```python
from build123d import *

# Parameters (mm, degrees)
PAD_DEPTH       = 8
PAD001_DEPTH    = 4
POCKET_DEPTH    = 5
SKETCH003_W     = 13
SKETCH003_H     = 7
PAD002_DEPTH    = 1
SKETCH004_R     = 0.5
POCKET001_DEPTH = 13.001
PAD003_DEPTH    = 14
PAD004_DEPTH    = 14
SKETCH007_R     = 1.5
PAD005_DEPTH    = 6
POCKET002_DEPTH = 5
SKETCH009_R     = 3
POCKET003_DEPTH = 15
SKETCH010_W     = 190
SKETCH010_H     = 10
POCKET004_DEPTH = 10
SKETCH011_W     = 40
SKETCH011_H     = 13
POCKET005_DEPTH = 3
PAD006_DEPTH    = 14
SKETCH014_W     = 25
SKETCH014_H     = 9
POCKET006_DEPTH = 15
SKETCH015_W     = 19.00002
SKETCH015_H     = 12
PAD007_DEPTH    = 1
SKETCH016_W     = 50
SKETCH016_H     = 9
PAD008_DEPTH    = 1
SKETCH017_W     = 3.141787
SKETCH017_H     = 1.901607
PAD009_DEPTH    = 2
SKETCH018_W     = 15
SKETCH018_H     = 8
POCKET007_DEPTH = 5
SKETCH019_W     = 4.140358
SKETCH019_H     = 3.938392
PAD010_DEPTH    = 1
FILLET_R        = 4


with BuildPart() as part:
    # Sketch → Pad (new body)
    with BuildSketch(Plane.XY):
        with BuildLine():
            Line((107.5, 0), (107.5, -35))
            Line((107.5, -35), (-107.5, -35))
            Line((-107.5, -35), (-107.5, 0))
            Line((-107.5, 0), (-0.930233, -9.956639))
            ThreePointArc((-0.930233, -9.956639), (0, -10), (0.930233, -9.956639))
            Line((0.930233, -9.956639), (107.5, 0))
        make_face()
    extrude(amount=PAD_DEPTH)

    # Sketch001 (on Face8 of Pad) → Pad001 (join)
    with BuildSketch(Plane.XY.offset(8)):
        with BuildLine():
            Line((107.5, 0), (107.5, -35))
            Line((107.5, -35), (-107.5, -35))
            Line((-107.5, -35), (-107.5, 0))
            Line((-107.5, 0), (-15, 0))
            Line((-15, 0), (-15, 2))
            ThreePointArc((15, 2), (0, 17), (-15, 2))
            Line((15, 2), (15, 0))
            Line((15, 0), (107.5, 0))
        make_face()
    extrude(amount=PAD001_DEPTH)

    # Sketch002 (on Face12 of Pad001) → Pocket (cut)
    with BuildSketch(Plane.XY.offset(12)):
        with BuildLine():
            ThreePointArc((3, -5.196152), (0, 6), (-3, -5.196152))
            Line((-3, -5.196152), (-3, -6.5))
            ThreePointArc((-3, -6.5), (0, -9.5), (3, -6.5))
            Line((3, -5.196152), (3, -6.5))
        make_face()
    extrude(amount=-POCKET_DEPTH, mode=Mode.SUBTRACT)

    # Sketch003 (on Face12 of Pocket) → Pad002 (join)
    with BuildSketch(Plane.XY.offset(12)):
        with Locations((0, 10)):
            Rectangle(SKETCH003_W, SKETCH003_H)
        with Locations((0, -20)):
            Rectangle(SKETCH003_W, SKETCH003_H)
    extrude(amount=PAD002_DEPTH)

    # Sketch004 (on Face31 of Pad002) → Pocket001 (cut, through all)
    with BuildSketch(Plane.XY.offset(13)):
        with Locations((0, 8.75)):
            Circle(SKETCH004_R)
        with Locations((0, -19.25)):
            Circle(SKETCH004_R)
    extrude(amount=-POCKET001_DEPTH, mode=Mode.SUBTRACT)

    # Sketch005 (on Face13 of Pocket001) → Pad003 (join)
    with BuildSketch(Plane.XY.offset(12)):
        with BuildLine():
            ThreePointArc((-6.5, 13.5), (-8.621333, 12.621327), (-9.50002, 10.5))
            Line((-9.50002, 10.5), (-9.50002, -20.5))
            ThreePointArc((-9.50002, -20.5), (-8.621333, -22.621327), (-6.5, -23.5))
            Line((-6.5, -23.5), (-6.5, 13.5))
        make_face()
        with BuildLine():
            ThreePointArc((6.5, -23.5), (8.62132, -22.62132), (9.5, -20.5))
            Line((9.5, 10.5), (9.5, -20.5))
            ThreePointArc((9.5, 10.5), (8.62132, 12.62132), (6.5, 13.5))
            Line((6.5, 13.5), (6.5, -23.5))
        make_face()
    extrude(amount=PAD003_DEPTH)

    # Sketch006 (on Face13 of Pad003) → Pad004 (join)
    with BuildSketch(Plane.XY.offset(12)):
        with BuildLine():
            Line((-107.5, 0), (-15, 0))
            Line((-15, 0), (-15, 2))
            ThreePointArc((15, 2), (0, 17), (-15, 2))
            Line((15, 0), (15, 2))
            Line((15, 0), (107.5, 0))
            Line((107.5, 0), (107.5, -2))
            Line((107.5, -2), (13, -2))
            Line((13, 2), (13, -2))
            ThreePointArc((13, 2), (0, 15), (-13, 2))
            Line((-13, 2), (-13, -2))
            Line((-13, -2), (-107.5, -2))
            Line((-107.5, -2), (-107.5, 0))
        make_face()
    extrude(amount=PAD004_DEPTH)

    # Sketch007 (on Face14 of Pad004) → Pad005 (join)
    with BuildSketch(Plane.XY.offset(12)):
        with BuildLine():
            ThreePointArc((-107.5, -5.999985), (-100.671578, -8.828432), (-103.5, -2))
            Line((-103.5, -2), (-107.5, -2))
            Line((-107.5, -2), (-107.5, -5.999985))
        make_face()
        with Locations((-103.5, -6)):
            Circle(SKETCH007_R, mode=Mode.SUBTRACT)
        with BuildLine():
            ThreePointArc((-67.854249, -35), (-70.5, -28), (-73.145751, -35))
            Line((-73.145751, -35), (-67.854249, -35))
        make_face()
        with Locations((-70.5, -32)):
            Circle(SKETCH007_R, mode=Mode.SUBTRACT)
    extrude(amount=PAD005_DEPTH)

    # Sketch008 (on Face60 of Pad005) → Pocket002 (cut)
    with BuildSketch(Plane.XY.offset(26)):
        Polygon((-10.113396, 8.978042), (-5.598833, 12.580972), (-5.598833, 8.367229), (-10.113396, 4.764299), align=None)
    extrude(amount=-POCKET002_DEPTH, mode=Mode.SUBTRACT)

    # Sketch009 (on Face14 of Pocket002) → Pocket003 (cut)
    with BuildSketch(Plane.XY.offset(12)):
        with Locations((-82.5, -20)):
            Circle(SKETCH009_R)
        with Locations((-49.5, -20)):
            Circle(SKETCH009_R)
        with Locations((-16.5, -20)):
            Circle(SKETCH009_R)
        with Locations((16.5, -20)):
            Circle(SKETCH009_R)
        with Locations((49.5, -20)):
            Circle(SKETCH009_R)
        with Locations((82.5, -20)):
            Circle(SKETCH009_R)
    extrude(amount=-POCKET003_DEPTH, mode=Mode.SUBTRACT)

    # Sketch010 (on Face20 of Pocket003) → Pocket004 (cut)
    with BuildSketch(Plane.XY.offset(12)):
        with Locations((0, -20)):
            Rectangle(SKETCH010_W, SKETCH010_H)
    extrude(amount=-POCKET004_DEPTH, mode=Mode.SUBTRACT)

    # Sketch011 (on Face20 of Pocket004) → Pocket005 (cut)
    with BuildSketch(Plane.XY.offset(12)):
        with Locations((-35, -8.5)):
            Rectangle(SKETCH011_W, SKETCH011_H)
    extrude(amount=-POCKET005_DEPTH, mode=Mode.SUBTRACT)

    # Sketch013 → Pad006 (join)
    with BuildSketch(Plane.XY.offset(12)):
        Polygon((104.5, -2), (107.5, -2), (107.5, -35), (-68.5, -35), (-68.5, -32), (104.5, -32), align=None)
    extrude(amount=PAD006_DEPTH)

    # Sketch014 (on Face20 of Pocket005) → Pocket006 (cut)
    with BuildSketch(Plane.XY.offset(12)):
        with Locations((-33.5, -8.5)):
            Rectangle(SKETCH014_W, SKETCH014_H)
    extrude(amount=-POCKET006_DEPTH, mode=Mode.SUBTRACT)

    # Sketch015 → Pad007 (join)
    with BuildSketch(Plane.XY.offset(12)):
        with Locations((-1e-05, -26.5)):
            Rectangle(SKETCH015_W, SKETCH015_H)
    extrude(amount=PAD007_DEPTH)

    # Sketch016 → Pad008 (join)
    with BuildSketch(Plane.XZ.offset(15)):
        with Locations((-34, 11.5)):
            Rectangle(SKETCH016_W, SKETCH016_H)
    extrude(amount=PAD008_DEPTH)

    # Sketch017 → Pad009 (join)
    with BuildSketch(Plane.XY):
        with Locations((0.426476, -19.263597)):
            Rectangle(SKETCH017_W, SKETCH017_H)
    extrude(amount=PAD009_DEPTH)

    # Sketch018 (on Face36 of Pad009) → Pocket007 (cut)
    with BuildSketch(Plane.XZ.offset(35)):
        with Locations((-61, 22)):
            Rectangle(SKETCH018_W, SKETCH018_H)
    extrude(amount=-POCKET007_DEPTH, mode=Mode.SUBTRACT)

    # Sketch019 (on Face7 of Pocket007) → Pad010 (join)
    with BuildSketch(Plane(origin=(0, 0, 8), x_dir=(1, 0, 0), z_dir=(0, 0, -1))):
        with Locations((0.364777, -8.489882)):
            Rectangle(SKETCH019_W, SKETCH019_H)
    extrude(amount=-PAD010_DEPTH)

    # Fillet
    fillet_edges = [part.edges().sort_by_distance(p)[0] for p in [
        (-46, -13, 4.5),
        (-21, -13, 4.5),
        (-21, -4, 8.5),
        (-46, -4, 8.5),
    ]]
    fillet(fillet_edges, radius=FILLET_R)


solid = part.part
```
Work out the finished part from the listing and answer in its coordinate system (mm). A direction names the side the tool comes from. Give positions to 0.01 mm unless a question says otherwise; leave off trailing zeros. Write each loop counter-clockwise with the first axis right and the second up, starting at its lowest first coordinate (ties: lowest second). Pieces come first, ordered by that corner, then holes.
(1) Flat-ended cylindrical pins translate along their axes: pin 1 Ø5 at (x, y) = (9.5, 10) entering from -Z; pin 2 Ø2 at (y, z) = (5.5, 19) entering from -X; pin 3 Ø6.5 at (x, y) = (-103, -7.5) entering from +Z. Find the tip coordinate at first contact, or state that the pin passes through.
Final values:
pin 1: stops at z = 8
pin 2: stops at x = -14.79
pin 3: stops at z = 18
(2) The mould has two halves that part along Y. Classify faces 6 (the flat face through (8, 1, 8)), 7 (the cylindrical face through (46.5, -19.9, 1)), 8 (the flat face through (-11.106, -9.006, 3.944)), 9 (the cylindrical face through (-0.1, -9.5, 10)): pulls with the +Y half, pulls with the -Y half, needs draft (parallel to the pull), parting line crosses it, or undercut.
Final values:
face 6: needs draft
face 7: undercut
face 8: pulls with the +Y half
face 9: undercut
(3) The part is cut by section B-B on x = 82.5. Write down the section's boundary in (y, z), plus the area to 3 significant figures.
Final values:
outline: (-35, 0) - (-23, 0) - (-23, 2) - (-25, 2) - (-25, 12) - (-32, 12) - (-32, 26) - (-35, 26) - close; (-17, 0) - (-2.34, 0) - (-2.34, 8) - (0, 8) - (0, 26) - (-2, 26) - (-2, 12) - (-15, 12) - (-15, 2) - (-17, 2) - close
area: 359 mm2
(4) The part is cut by section A-A on x = -49.5. Write down the section's boundary in (y, z).
Final values:
outline: (-35, 0) - (-23, 0) - (-23, 2) - (-25, 2) - (-25, 12) - (-32, 12) - (-32, 26) - (-35, 26) - close; (-17, 0) - (-5.42, 0) - (-5.42, 8) - (0, 8) - (0, 26) - (-2, 26) - (-2, 9) - (-15, 9) - (-15, 16) - (-16, 16) - (-16, 7) - (-15, 7) - (-15, 2) - (-17, 2) - close
(5) Straight lines are drawn through the part: line 1 (X direction, y = -12, z = 17.25); line 2 (Y direction, x = 35.5, z = 13); line 3 (Y direction, x = -34.5, z = 2.25). For each, find the intervals that lie inside material, in ascending order.
Final values:
line 1: x = -9.5 to -6.5, 6.5 to 9.5, 104.5 to 107.5
line 2: y = -35 to -32, -2 to 0
line 3: y = -35 to -25, -15 to -13
(6) Which of the six approach directions +Z, -Z, +X, -X, +Y, -Y give full straight-line access (tool end or side, diameter ignored) to faces 1 (the flat face through (-105.3, -5.9, 18)), 2 (the cylindrical face through (-45.644, -6.349, 5.437)), 3 (the flat face through (53.469, -5.048, 3.944)), 4 (the cylindrical face through (0, 17, 17)), 5 (the flat face through (-35, -14, 9))?
Final values:
face 1: +Z, -X, -Y
face 2: +Z, -Z
face 3: -Z, +Y
face 4: +Z, -Z, +Y
face 5: +Z
